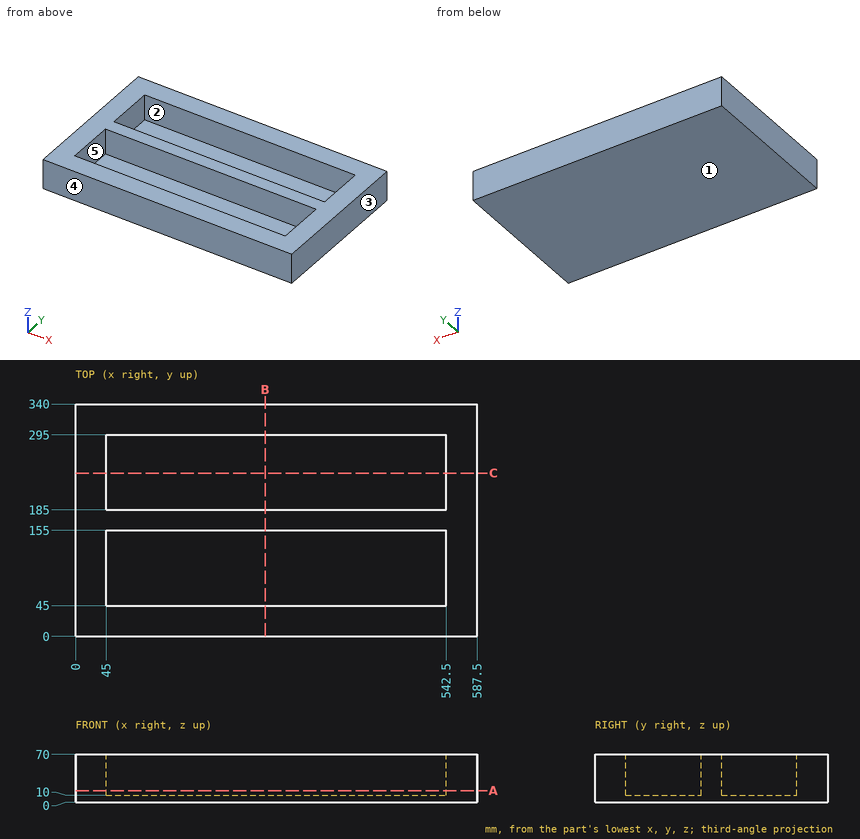
Verification items for this drawing (mm, ordinates from the low corner). A direction names the side the tool comes from. Round coordinates to 2 decimals unless told otherwise and drop trailing zeros. Write each loop counter-clockwise with the first axis right and the second up, starting at its lowest first coordinate (ties: lowest second). Pieces come first, ordered by that corner, then holes. Notation, with made-up numbers: (55, 35.25) - (99, 35.25) arc R12 cw to (99, 56.25) - close; hole circle Ø2 at (-22, -11.75). An arc over 180 degrees is marked (long way). One line per item, written item: value.
1. Depth check by flat-ended pin: pin 1 Ø2 at (x, y) = (267.5, 236) entering from +Z. Enter the tip coordinate at first touch or a pass-through.
The answers:
pin 1: stops at z = 10
2. Mould release check, pull along Y, two halves, no side actions. Record for the marked faces 3, 4 and 5: released by +Y, released by -Y, zero draft, split by the parting line, or undercut.
The answers:
face 3: zero draft
face 4: released by -Y
face 5: undercut
3. Cross-section at B-B on x = 277.5. Record the boundary of the cut face in (y, z), and give its area (3 significant figures).
The answers:
outline: (0, 0) - (340, 0) - (340, 70) - (295, 70) - (295, 10) - (185, 10) - (185, 70) - (155, 70) - (155, 10) - (45, 10) - (45, 70) - (0, 70) - close
area: 10,600 mm^2
4. Set-up check for the marked faces 1 and 2: record each of +Z, -Z, +X, -X, +Y, -Y from which the full face is reachable in a straight line by a thin tool's end or side.
The answers:
face 1: -Z, +X, -X, +Y, -Y
face 2: +Z
5. Scan lines: L1, parallel to Y at x = 402, z = 43; L2, parallel to X at y = 258, z = 63; L3, parallel to Z at x = 355, y = 154. Record each from-to range of solid material in increasing order.
The answers:
L1: y = 0 to 45, 155 to 185, 295 to 340
L2: x = 0 to 45, 542.5 to 587.5
L3: z = 0 to 10
6. Cross-section at C-C on y = 239. Record the boundary of the cut face in (x, z), and give its area (3 significant figures).
The answers:
outline: (0, 0) - (587.5, 0) - (587.5, 70) - (542.5, 70) - (542.5, 10) - (45, 10) - (45, 70) - (0, 70) - close
area: 11,300 mm^2
7. Cross-section at A-A on z = 17. Record the boundary of the cut face in (x, y), and give its area (3 significant figures).
The answers:
outline: (0, 0) - (587.5, 0) - (587.5, 340) - (0, 340) - close; hole (45, 45) - (542.5, 45) - (542.5, 155) - (45, 155) - close; hole (45, 185) - (542.5, 185) - (542.5, 295) - (45, 295) - close
area: 90,300 mm^2
